Verification items for the finished model (mm, model axes). A direction names the side the tool comes from. Round coordinates to 2 decimals unless told otherwise and drop trailing zeros. Order: outer loops, then holes, each group sorted by start corner. A loop starts at its lowest first (then second) coordinate and runs counter-clockwise, first axis right, second up. Notation, with made-up numbers: (11, -37.75) -> (34, -37.75) arc R5 cw to (34, -31.75) -> close; hole circle Ø5 at (73, -6). An arc over 180 degrees is marked (long way). Return JSON: item names as keys, results as strings. Group by question number.
Item 1: Draft check along X on faces 1 (the cylindrical face through (-25.362, 17.644, 7.889)), 2 (the flat face through (25, -31.75, 8)), 3 (the flat face through (-22, -26.162, 8)). Enter one of: pulls with the +X half, pulls with the -X half, needs draft (parallel to the pull), parting line crosses it, or undercut.
Item 2: Sectioned sample at A-A on x = 0. Record the cut outline in (y, z).
Item 3: Sectioned sample at B-B on z = 13.5. Record the cut outline in (x, y) (3 decimals), plus the area to 3 significant figures.
Item 4: Depth check by flat-ended pin: pin 1 Ø3 at (x, z) = (-9, 10) entering from -Y; pin 2 Ø7 at (y, z) = (34, 11.5) entering from +X; pin 3 Ø7 at (y, z) = (34.5, 7.5) entering from -X. Enter the tip coordinate at first touch or a pass-through.
Item 5: Sectioned sample at C-C on y = 26.5. Record the cut outline in (x, z), plus the area to 3 significant figures.
Item 6: Access from +Z, -Z, +X, -X, +Y, -Y to the whole of each face (thin tool, end or side, straight path). Record for faces 4 (the flat face through (-24.635, -13, 8)), 5 (the flat face through (-19.05, -29, 8)), 6 (the flat face through (-7.874, 35, 8)).
Item 7: Scan lines: probe 1 along X at (y, z) = (-19, 4.5); probe 2 along Z at (x, y) = (0, 31.5); probe 3 along X at (y, z) = (33, 2). Record each from-to range of solid material in increasing order. Write a range as from..to.
Item 8: Sectioned sample at D-D on z = 9. Record the cut outline in (x, y) (3 decimals).
```python
from build123d import *

# Parameters (mm, degrees)
BOSS_EXTRUDE1_DEPTH      = 16.002
FILLET1_R                = 3.175
F_5_16_18_TAPPED_HOLE1_D = 6.5278


with BuildPart() as part:
    # Sketch2 → Boss-Extrude1 (new body)
    with BuildSketch(Plane.XY):
        with BuildLine():
            Line((-24.634929355, 0), (-24.634929355, -26.162))
            Line((-24.634929355, -26.162), (-19.05, -26.162))
            Line((-19.05, -26.162), (-19.05, -31.75))
            Line((-19.05, -31.75), (-30.988, -31.75))
            Line((-30.988, -31.75), (-30.988, 0))
            ThreePointArc((-30.988, 0), (-24.5240996, 18.768520453), (-7.874, 29.576552267))
            Line((-7.874, 29.576552267), (-7.874, 38.1))
            Line((-7.874, 38.1), (7.874, 38.1))
            Line((7.874, 38.1), (7.874, 29.576552267))
            ThreePointArc((7.874, 29.576552267), (24.5240996, 18.768520453), (30.988, 0))
            Line((30.988, 0), (30.988, -31.75))
            Line((30.988, -31.75), (19.05, -31.75))
            Line((19.05, -31.75), (19.05, -26.162))
            Line((19.05, -26.162), (24.634929355, -26.162))
            Line((24.634929355, -26.162), (24.634929355, 0))
            ThreePointArc((24.634929355, 0), (0, 24.634929355), (-24.634929355, 0))
        make_face()
    extrude(amount=BOSS_EXTRUDE1_DEPTH)

    # Fillet1
    fillet1_edges = [part.edges().sort_by_distance(p)[0] for p in [
        (-7.874, 29.576552267, 8.001),
        (7.874, 29.576552267, 8.001),
    ]]
    fillet(fillet1_edges, radius=FILLET1_R)

    # 5/16-18 Tapped Hole1 (through all)
    with Locations(Plane(origin=(0, 38.1, 0), x_dir=(1, 0, 0), z_dir=(0, 1, 0))):
        with Locations((0, -8.001)):
            Hole(F_5_16_18_TAPPED_HOLE1_D / 2)


solid = part.part
```
Recorded:
{
 "1": {"face 1": "pulls with the -X half", "face 2": "needs draft", "face 3": "undercut"},
 "2": {"outline": "(24.63, 0) -> (38.1, 0) -> (38.1, 4.74) -> (24.63, 4.74) -> close; (24.63, 11.26) -> (38.1, 11.26) -> (38.1, 16) -> (24.63, 16) -> close"},
 "3": {"outline": "(-30.988, -31.75) -> (-19.05, -31.75) -> (-19.05, -26.162) -> (-24.635, -26.162) -> (-24.635, 0) arc R24.635 cw to (24.635, 0) -> (24.635, -26.162) -> (19.05, -26.162) -> (19.05, -31.75) -> (30.988, -31.75) -> (30.988, 0) arc R30.48 ccw to (10.055, 28.946) arc R3.175 cw to (7.874, 31.962) -> (7.874, 38.1) -> (-7.874, 38.1) -> (-7.874, 31.962) arc R3.175 cw to (-10.055, 28.946) arc R30.48 ccw to (-30.988, 0) -> close", "area": "1,130 mm²"},
 "4": {"pin 1": "y = 22.29", "pin 2": "x = 8.23", "pin 3": "x = -8.02"},
 "5": {"outline": "(-15.57, 0) -> (15.57, 0) -> (15.57, 16) -> (-15.57, 16) -> close; hole circle Ø6.53 at (0, 8)", "area": "465 mm²"},
 "6": {"face 4": "+Z, -Z", "face 5": "+Z, -Z, -Y", "face 6": "+Z, -Z, -X, +Y"},
 "7": {"probe 1": "-30.99..-24.63, 24.63..30.99", "probe 2": "0..4.74, 11.26..16", "probe 3": "-7.87..7.87"},
 "8": {"outline": "(-30.988, -31.75) -> (-19.05, -31.75) -> (-19.05, -26.162) -> (-24.635, -26.162) -> (-24.635, 0) arc R24.635 cw to (-3.107, 24.438) -> (-3.107, 38.1) -> (-7.874, 38.1) -> (-7.874, 31.962) arc R3.175 cw to (-10.055, 28.946) arc R30.48 ccw to (-30.988, 0) -> close; (3.107, 24.438) arc R24.635 cw to (24.635, 0) -> (24.635, -26.162) -> (19.05, -26.162) -> (19.05, -31.75) -> (30.988, -31.75) -> (30.988, 0) arc R30.48 ccw to (10.055, 28.946) arc R3.175 cw to (7.874, 31.962) -> (7.874, 38.1) -> (3.107, 38.1) -> close"}
}
